For this review, use the dimensioned drawing (mm, ordinates from the lowest corner) and the shaded views. A direction names the side the tool comes from. Round coordinates to 2 decimals unless told otherwise and drop trailing zeros. Order: outer loops, then holes, each group sorted by start corner. A loop starts at its lowest first (then second) coordinate and runs counter-clockwise, first axis right, second up. Notation, with made-up numbers: M 70,13.25 L 87,13.25 A30 cw 87,48.25 Z; hole C 38.25,68.25 d11. An arc over 180 degrees is marked long. Put each result on its own line as item: value.
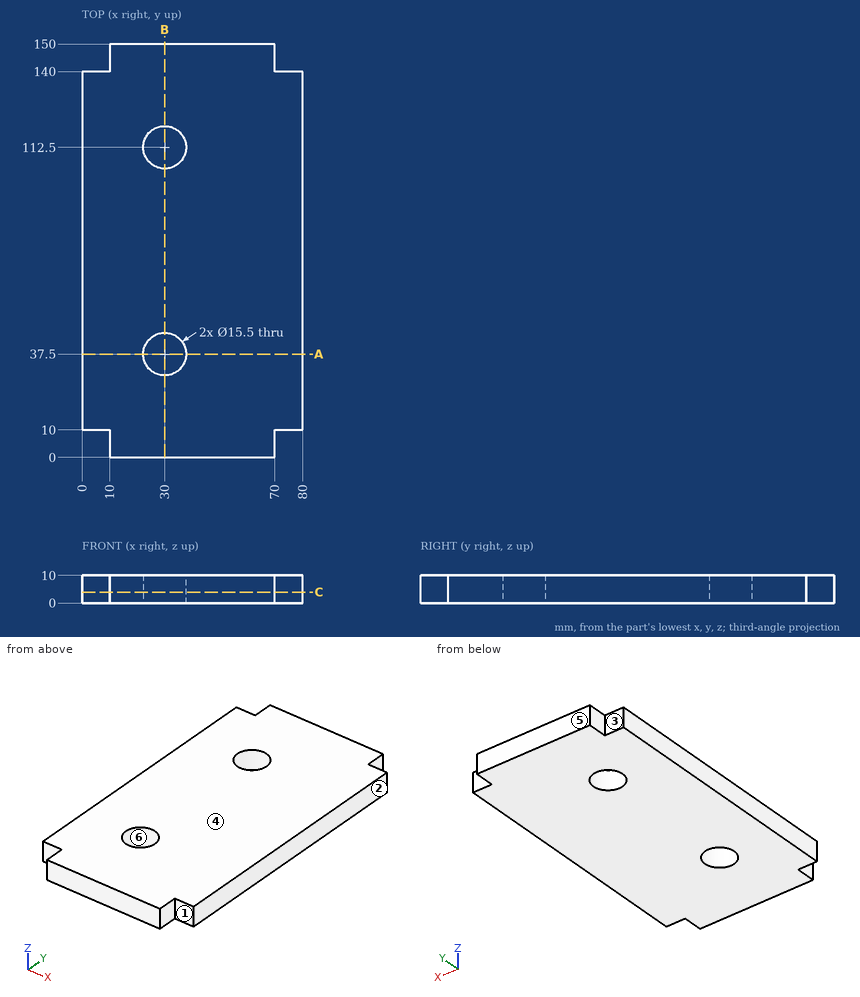
(1) Insertion check: pin 1 Ø5 at (x, z) = (75.5, 6.5) entering from +Y; pin 2 Ø5 at (y, z) = (144, 5.5) entering from -X; pin 3 Ø25 at (x, y) = (30, 112.5) entering from +Z; pin 4 Ø12.5 at (x, y) = (30, 37.5) entering from -Z. Each pin has a flat end and moves straight along its axis. Give the tip position at first contact, or say it passes through.
A:
pin 1: stops at y = 140
pin 2: stops at x = 10
pin 3: stops at z = 10
pin 4: passes through
(2) Add section B-B on x = 30. Give the boundary of the cut face in (y, z).
A:
outline: M 0,0 L 29.75,0 L 29.75,10 L 0,10 Z; M 45.25,0 L 104.75,0 L 104.75,10 L 45.25,10 Z; M 120.25,0 L 150,0 L 150,10 L 120.25,10 Z
(3) Add section A-A on y = 37.5. Give the boundary of the cut face in (x, z).
A:
outline: M 0,0 L 22.25,0 L 22.25,10 L 0,10 Z; M 37.75,0 L 80,0 L 80,10 L 37.75,10 Z
(4) For the marked faces 1, 2 and 3, list the 3-axis set-ups (+Z, -Z, +X, -X, +Y, -Y) from which the entire face can be reached by the end or side of a thin tool; tool diameter is ignored.
A:
face 1: +Z, -Z, +X, -Y
face 2: +Z, -Z, +X, +Y, -Y
face 3: +Z, -Z, -X, +Y
(5) To check wall thickness, follow L1, parallel to Y at x = 30, z = 4.5; L2, parallel to X at y = 37.5, z = 3.25; L3, parallel to Y at x = 75.5, z = 6.5. State the ranges of each line that lie inside material, in increasing order.
A:
L1: y = 0 to 29.75, 45.25 to 104.75, 120.25 to 150
L2: x = 0 to 22.25, 37.75 to 80
L3: y = 10 to 140
(6) Draft analysis for pull direction Y (two halves, no side actions). For the marked faces 4, 5 and 6, state which applies: released by +Y, released by -Y, zero draft, split by the parting line, or undercut.
A:
face 4: zero draft
face 5: released by +Y
face 6: undercut
(7) Add section C-C on z = 4. Give the boundary of the cut face in (x, y).
A:
outline: M 0,10 L 10,10 L 10,0 L 70,0 L 70,10 L 80,10 L 80,140 L 70,140 L 70,150 L 10,150 L 10,140 L 0,140 Z; hole C 30,37.5 d15.5; hole C 30,112.5 d15.5
